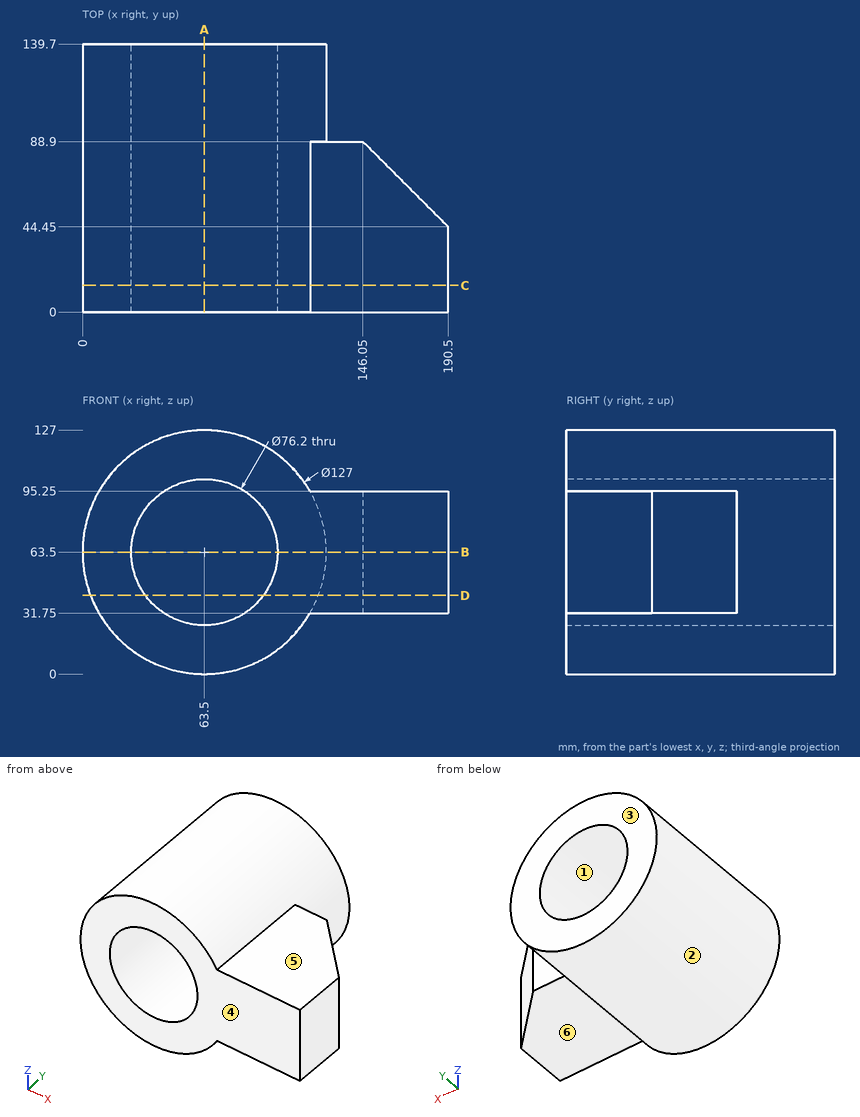
Geometry: see drawing. Coordinates: mm, zero at the bounding-box minimum. A direction names the side the tool comes from. Coordinates: 2 decimals unless noted, no trailing zeros. Loops run counter-clockwise (first coordinate to the right, second up) from the corner with the lowest first, then second, coordinate; pieces in that order, holes last. Notation, with made-up numbers: (-12.75, 46.25) -> (10.25, 46.25) arc R28 cw to (10.25, 74.25) -> close; hole circle Ø1 at (-17, 11). An arc over 180 degrees is marked (long way). Use a Markdown table: item, result.
1) Contact query for flat-ended pins moving along their axis: pin 1 (1.5 mm diameter, centred on x = 28, z = 72.5, fed in from +Y); pin 2 (10 mm diameter, centred on x = 115, y = 66.5, fed in from -Z); pin 3 (8 mm diameter, centred on y = 81.5, z = 37.5, fed in from -X); pin 4 (5 mm diameter, centred on y = 58, z = 113, fed in from +X). Output: stop coordinate, or through.
Results found:
| item | result |
|---|---|
| pin 1 | passes through |
| pin 2 | stops at z = 20.26 |
| pin 3 | stops at x = 3.93 |
| pin 4 | stops at x = 106.2 |
2) Cut plane A-A (x = 63.5). Return the cut outline in (y, z).
Results found:
| item | result |
|---|---|
| outline | (0, 0) -> (139.7, 0) -> (139.7, 25.4) -> (0, 25.4) -> close; (0, 101.6) -> (139.7, 101.6) -> (139.7, 127) -> (0, 127) -> close |
3) Cut plane C-C (y = 14). Return the cut outline in (x, z).
Results found:
| item | result |
|---|---|
| outline | (118.49, 31.75) -> (190.5, 31.75) -> (190.5, 95.25) -> (118.49, 95.25) arc R63.5 ccw (long way) to start; hole circle Ø76.2 at (63.5, 63.5) |
4) Material intervals for line 1 along X through (y, z) = (104, 63.5); line 2 along X through (y, z) = (44, 63), sorted ascending. Write a range as from..to.
Results found:
| item | result |
|---|---|
| line 1 | x = 0..25.4, 101.6..127 |
| line 2 | x = 0..25.4, 101.6..190.5 |
5) Pull-direction query (X, two-part tool) for the marked faces 1, 2 and 3; classes: released by +X, released by -X, zero draft, split by the parting line, or undercut.
Results found:
| item | result |
|---|---|
| face 1 | undercut |
| face 2 | split by the parting line |
| face 3 | zero draft |
6) Cut plane D-D (z = 41). Return the cut outline in (x, y).
Results found:
| item | result |
|---|---|
| outline | (4.12, 0) -> (32.75, 0) -> (32.75, 139.7) -> (4.12, 139.7) -> close; (94.25, 0) -> (190.5, 0) -> (190.5, 44.45) -> (146.05, 88.9) -> (122.88, 88.9) -> (122.88, 139.7) -> (94.25, 139.7) -> close |
7) Access query for the marked faces 4, 5 and 6. Directions: +Z, -Z, +X, -X, +Y, -Y. A direction counts if a zero-diameter tool reaches every point of the face in a straight line with its end or side. Return the directions, or none.
Results found:
| item | result |
|---|---|
| face 4 | +Z, -Z, +X, -X, -Y |
| face 5 | +Z, +X, +Y, -Y |
| face 6 | -Z, +X, +Y, -Y |
8) Cut plane B-B (z = 63.5). Return the cut outline in (x, y), then the cut area to 3 significant figures.
Results found:
| item | result |
|---|---|
| outline | (0, 0) -> (25.4, 0) -> (25.4, 139.7) -> (0, 139.7) -> close; (101.6, 0) -> (190.5, 0) -> (190.5, 44.45) -> (146.05, 88.9) -> (127, 88.9) -> (127, 139.7) -> (101.6, 139.7) -> close |
| area | 11,800 mm2 |
